For this review, take the finished solid that the model builds, in its own axes (mm). Face numbers are marked on the shaded views. Coordinates: 2 decimals unless noted, no trailing zeros. Write each loop counter-clockwise with the first axis right and the second up, starting at its lowest first coordinate (ties: lowest second). Pieces come first, ordered by that corner, then holes. Notation, with made-up numbers: M 10.5,5 L 45.5,5 A9 ccw 45.5,19 Z; hole C 51.25,6.25 d6. An arc over 180 degrees is marked long. Return JSON: item names as keys, results as strings.
Autodesk Inventor part; units mm, degrees
ref_plane "YZ Plane" through (0, 0, 0) normal (1, 0, 0) x (0, 1, 0)
ref_plane "XZ Plane" through (0, 0, 0) normal (0, 1, 0) x (-1, 0, 0)
ref_plane "XY Plane" through (0, 0, 0) normal (0, 0, 1) x (1, 0, 0)
sketch "Sketch1" plane through (0, 0, 0) normal (0, 1, 0) x (-1, 0, 0)
  line L0 (101.8, 101.8) -> (-101.8, 101.8)
  line L1 (-101.8, 101.8) -> (-101.8, -91.8)
  line L2 (-101.8, -91.8) -> (101.8, -91.8)
  line L3 (101.8, -91.8) -> (101.8, 101.8)
  point P0 (0, 101.8)
  point P1 (101.8, 5)
  dimension "d0" = 203.6
  dimension "d1" = 193.6
extrude "Plate1" add sketch "Sketch1" along normal blind 0.5
sketch "Sketch2" plane through (0, 0.5, 0) normal (0, 1, 0) x (1, 0, 0)
  line L0 (-52.5, -52.5) -> (52.5, 52.5) construction
  line L1 (52.5, -52.5) -> (-52.5, 52.5) construction
  point P0 (0, 0)
  point P1 (0, 0)
  dimension "d7" = 105
  dimension "d8" = 105
hole "Hole1" at (-52.5, 0.5, 52.5) at (-52.5, 0.5, -52.5) at (52.5, 0.5, 52.5) at (52.5, 0.5, -52.5) direction (0, -1, 0) diameter 6 depth 0.5 tip angle 118
sketch "Sketch3" plane through (0, 0.5, 0) normal (0, 1, 0) x (1, 0, 0)
  line L0 (-60, -60) -> (60, -60)
  line L1 (60, -60) -> (60, 60)
  line L2 (60, 60) -> (-60, 60)
  line L3 (-60, 60) -> (-60, -60)
  arc A0 (-60, -20.7906) -> (-20.7906, -60) centre (0, 0) ccw
  arc A1 (20.7906, -60) -> (60, -20.7906) centre (0, 0) ccw
  arc A2 (60, 20.7906) -> (20.7906, 60) centre (0, 0) ccw
  arc A3 (-20.7906, 60) -> (-60, 20.7906) centre (0, 0) ccw
  point P0 (0, -48.7613)
  point P1 (-70.0637, 0)
  point P2 (-60, 0)
  point P3 (0, -60)
  dimension "d17" = 120
extrude "Cut1" cut sketch "Sketch3" against normal blind 0.5 contours A0 L3 A3 L2 A2 L1 A1 L0
equation "\"d8\" = d7"
equation "\"d14\" = Thickness"
equation "\"d19\" = Thickness"
equation "\"d2\" = Thickness"
equation "\"BendRadius\" = Thickness"
equation "\"BendReliefWidth\" = Thickness"
equation "\"BendReliefDepth\" = 0.5 * Thickness"
equation "\"CornerReliefSize\" = 4 * Thickness"
equation "\"MinimumRemnant\" = 2 * Thickness"
equation "\"TransitionRadius\" = BendRadius"
equation "\"JacobiRadiusSize\" = BendRadius"
equation "\"GapSize\" = Thickness"
properties part number "top panel" material "Stainless Steel"
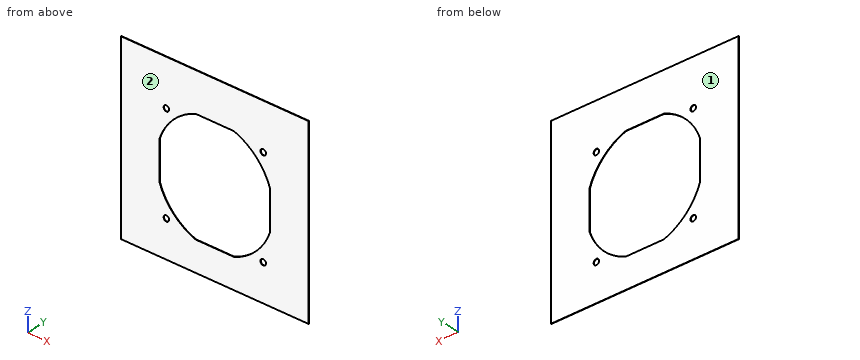
1. We need section C-C (y = 0.35). State the section outline as (x, z) points.
Checks:
{"outline": "M -101.8,-91.8 L 101.8,-91.8 L 101.8,101.8 L -101.8,101.8 Z; hole M -60,-20.79 A63.5 ccw -20.79,-60 L 20.79,-60 A63.5 ccw 60,-20.79 L 60,20.79 A63.5 ccw 20.79,60 L -20.79,60 A63.5 ccw -60,20.79 Z; hole C -52.5,-52.5 d6; hole C -52.5,52.5 d6; hole C 52.5,-52.5 d6; hole C 52.5,52.5 d6"}
2. We need section D-D (z = 52.5). State the section outline as (x, y) points, plus the area to 3 significant figures.
Checks:
{"outline": "M -101.8,0 L -55.5,0 L -55.5,0.5 L -101.8,0.5 Z; M -49.5,0 L -35.72,0 L -35.72,0.5 L -49.5,0.5 Z; M 35.72,0 L 49.5,0 L 49.5,0.5 L 35.72,0.5 Z; M 55.5,0 L 101.8,0 L 101.8,0.5 L 55.5,0.5 Z", "area": "60.1 mm2"}
3. We need section B-B (x = 8). State the section outline as (y, z) points, plus the area to 3 significant figures.
Checks:
{"outline": "M 0,-91.8 L 0.5,-91.8 L 0.5,-60 L 0,-60 Z; M 0,60 L 0.5,60 L 0.5,101.8 L 0,101.8 Z", "area": "36.8 mm2"}
4. Draft analysis for pull direction Y (two halves, no side actions). For the marked faces 1 and 2, state which applies: +Y half, -Y half, draft (parallel to the pull), parting line (faces both ways), or undercut.
Checks:
{"face 1": "+Y half", "face 2": "-Y half"}
5. We need section A-A (z = -15.5). State the section outline as (x, y) points, plus the area to 3 significant figures.
Checks:
{"outline": "M -101.8,0 L -60,0 L -60,0.5 L -101.8,0.5 Z; M 60,0 L 101.8,0 L 101.8,0.5 L 60,0.5 Z", "area": "41.8 mm2"}
6. Clearance check with a flat-ended pin moving along its axis: pin 1 Ø5 at (x, z) = (52.5, -52.5) entering from -Y. State where the tip first meets the part, or that it passes through.
Checks:
{"pin 1": "through"}
7. Wall thickness on L1, parallel to X at y = 0.2, z = -18; L2, parallel to Z at x = 52.5, y = 0.1; L3, parallel to X at y = 0.4, z = -55: over which ranges is each line inside the solid? List them lowest first. Write a range as from..to.
Checks:
{"L1": "-101.8..-60, 60..101.8", "L2": "-91.8..-55.5, -49.5..-35.72, 35.72..49.5, 55.5..101.8", "L3": "-101.8..-54.16, -50.84..-31.74, 31.74..50.84, 54.16..101.8"}
